from build123d import *

# Parameters (mm, degrees)
F1_DEPTH = 5
F2_R     = 1
F3_R     = 1


with BuildPart() as f1:
    # F0 (on Front) → F1 (new body)
    with BuildSketch(Plane.XZ):
        Polygon((0, 60), (0, 0), (23, 0), (23, 38), (15, 38), (15, 60), align=None)
    extrude(amount=F1_DEPTH)

    # F2
    f2_edges = [f1.edges().sort_by_distance(p)[0] for p in [
        (0, -2.5, 60),
        (15, -2.5, 60),
        (23, -2.5, 38),
        (0, -2.5, 0),
        (23, -2.5, 0),
    ]]
    fillet(f2_edges, radius=F2_R)

    # F3
    f3_edges = [f1.edges().sort_by_distance(p)[0] for p in [
        (15, -2.5, 38),
    ]]
    fillet(f3_edges, radius=F3_R)


solid = f1.part
Verification items for the finished model (mm, model axes). A direction names the side the tool comes from. Round coordinates to 2 decimals unless told otherwise and drop trailing zeros. Loops run counter-clockwise (first coordinate to the right, second up) from the corner with the lowest first, then second, coordinate; pieces in that order, holes last. Notation, with made-up numbers: M 87,44.5 L 108,44.5 A12 ccw 108,55.5 Z; hole C 18.5,76.5 d9. An arc over 180 degrees is marked long. Write each question's results on one line, items separated by ' | '.
1) Section check A-A on y = -3. Record the boundary of the cut face in (x, z).
Checks:
outline: M 0,1 A1 ccw 1,0 L 22,0 A1 ccw 23,1 L 23,37 A1 ccw 22,38 L 16,38 A1 cw 15,39 L 15,59 A1 ccw 14,60 L 1,60 A1 ccw 0,59 Z
2) Scan lines: L1, parallel to X at y = -0.4, z = 39; L2, parallel to Z at x = 18, y = -0.3. Record each from-to range of solid material in increasing order. Write a range as from..to.
Checks:
L1: x = 0..15 | L2: z = 0..38
3) Access from +Z, -Z, +X, -X, +Y, -Y to the whole of each face (thin tool, end or side, straight path). Record for faces 4 (the flat face through (19, -2, 38)), 5 (the cylindrical face through (0.285, -2.535, 0.301)).
Checks:
face 4: +Z, +X, +Y, -Y | face 5: -Z, -X, +Y, -Y
4) Section check B-B on z = 48. Record the boundary of the cut face in (x, y), then the cut area to 3 significant figures.
Checks:
outline: M 0,-5 L 15,-5 L 15,0 L 0,0 Z | area: 75.0 mm2
5) Mould release check, pull along Z, two halves, no side actions. Record for faces 1 (the cylindrical face through (0.285, -2.535, 59.699)), 2 (the flat face through (0, -2, 30)), 3 (the flat face through (11, -2, 0)): released by +Z, released by -Z, zero draft, split by the parting line, or undercut.
Checks:
face 1: released by +Z | face 2: zero draft | face 3: released by -Z
